The drawing under review shows one solid part. Ordinate dimensions are in mm from its lowest x, y, z. Give positions to 0.01 mm unless a question says otherwise; leave off trailing zeros. Order: outer loops, then holes, each group sorted by start corner. A loop starts at its lowest first (then second) coordinate and runs counter-clockwise, first axis right, second up. Notation, with made-up numbers: M 85.5,69.25 L 133.5,69.25 A14 ccw 133.5,82.25 Z; hole C -13.5,33.5 d6. An arc over 180 degrees is marked long. Put each result on its own line as item: value. Start each with the question number.
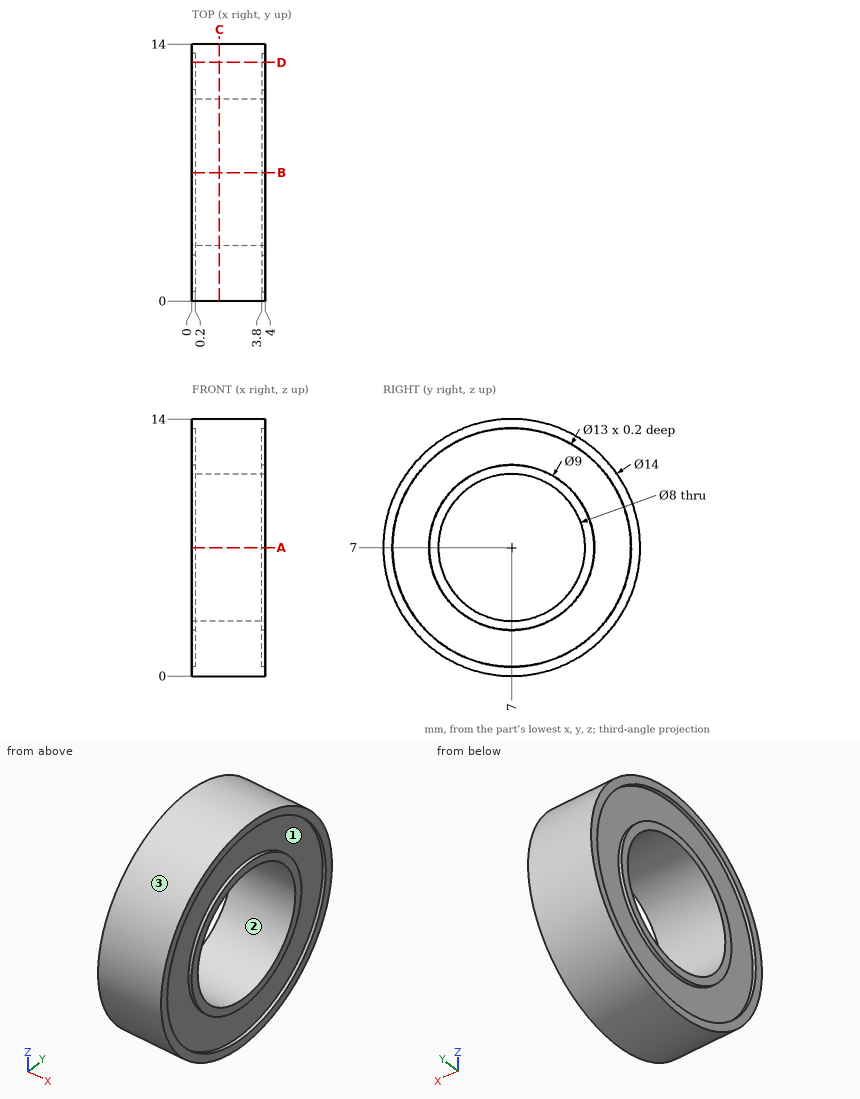
1. Consider section A-A on z = 7. Give the boundary of the cut face in (x, y), then the cut area to 3 significant figures.
2. Consider section D-D on y = 13. Give the boundary of the cut face in (x, z), then the cut area to 3 significant figures.
3. To check wall thickness, follow probe 1 along Y at (x, z) = (0.1, 7); probe 2 along Y at (x, z) = (0.25, 7); probe 3 along X at (y, z) = (1.5, 9.5). State the ranges of each line that lie inside material, in increasing order.
4. Consider section C-C on x = 1.5. Give the boundary of the cut face in (y, z).
5. The part is to be moulded in two halves that separate along Y. For the marked faces 1, 2 and 3, say which applies: +Y half, -Y half, draft (parallel to the pull), parting line (faces both ways), or undercut.
6. Insertion check: pin 1 (2 mm diameter, centred on x = 3.5, z = 5, fed in from +Y); pin 2 (2 mm diameter, centred on x = 1, z = 10, fed in from +Y). Each pin has a flat end and moves straight along its axis. Give the tip position at first contact, or say it passes through.
Returned:
1. outline: M 0,0 L 4,0 L 4,0.5 L 3.8,0.5 L 3.8,2.5 L 4,2.5 L 4,3 L 0,3 L 0,2.5 L 0.2,2.5 L 0.2,0.5 L 0,0.5 Z; M 0,11 L 4,11 L 4,11.5 L 3.8,11.5 L 3.8,13.5 L 4,13.5 L 4,14 L 0,14 L 0,13.5 L 0.2,13.5 L 0.2,11.5 L 0,11.5 Z
1. area: 22.4 mm2
2. outline: M 0,3.39 L 4,3.39 L 4,4.5 L 3.8,4.5 L 3.8,9.5 L 4,9.5 L 4,10.61 L 0,10.61 L 0,9.5 L 0.2,9.5 L 0.2,4.5 L 0,4.5 Z
2. area: 26.8 mm2
3. probe 1: y = 0 to 0.5, 2.5 to 3, 11 to 11.5, 13.5 to 14
3. probe 2: y = 0 to 3, 11 to 14
3. probe 3: x = 0.2 to 3.8
4. outline: C 7,7 d14; hole C 7,7 d8
5. face 1: undercut
5. face 2: undercut
5. face 3: parting line
6. pin 1: stops at y = 13.93
6. pin 2: stops at y = 13.71
